Geometry: final body of the model. Coordinates: model frame, mm. Face numbers are marked on the shaded views. A direction names the side the tool comes from. Round coordinates to 2 decimals unless told otherwise and drop trailing zeros. Loops run counter-clockwise (first coordinate to the right, second up) from the corner with the lowest first, then second, coordinate; pieces in that order, holes last. Notation, with made-up numbers: M 15,51.25 L 49,51.25 A34 ccw 49,84.25 Z; hole C 83,-17 d5. An arc over 180 degrees is marked long. Answer as a JSON object with one key per item and string values.
from build123d import *

# Parameters (mm, degrees)
F1_DEPTH = 25.4
F2_R     = 7.6978943935
F3_DEPTH = 25.4
F5_DEPTH = 25.4
F7_DEPTH = 12.7
F9_DEPTH = 12.7


with BuildPart() as f1:
    # F0 (on Front) → F1 (new body)
    with BuildSketch(Plane.XZ):
        Polygon((-11.8255742339, 38.1), (-37.2255742339, 38.1), (-37.2255742339, 0), (32.6244257661, 0), (32.6244257661, 12.7), (-11.8255742339, 12.7), align=None)
    extrude(amount=F1_DEPTH)

    # F2 (on face) → F3 (cut)
    with BuildSketch(Plane.XZ.offset(25.4)):
        with Locations((-24.5255742339, 25.4)):
            Circle(F2_R)
    extrude(amount=-F3_DEPTH, mode=Mode.SUBTRACT)

    # F4 (on face) → F5 (cut)
    with BuildSketch(Plane.XZ.offset(25.4)):
        with BuildLine():
            ThreePointArc((-37.2255742339, 30.0844254155), (-34.376772158, 35.2511979241), (-29.2099996494, 38.1))
            Line((-29.2099996494, 38.1), (-37.2255742339, 38.1))
            Line((-37.2255742339, 38.1), (-37.2255742339, 30.0844254155))
        make_face()
        with BuildLine():
            Line((-11.8255742339, 38.1), (-20.5647205525, 38.1))
            ThreePointArc((-20.5647205525, 38.1), (-14.8369913494, 35.0885828844), (-11.8255742339, 29.3608536814))
            Line((-11.8255742339, 29.3608536814), (-11.8255742339, 38.1))
        make_face()
    extrude(amount=-F5_DEPTH, mode=Mode.SUBTRACT)

    # F6 (on face) → F7 (cut)
    with BuildSketch(Plane.XY.offset(12.7)):
        with BuildLine():
            ThreePointArc((26.2744257661, -12.7), (24.4145538267, -8.2098719395), (19.9244257661, -6.35))
            ThreePointArc((19.9244257661, -6.35), (13.5744257661, -12.7), (19.9244257661, -19.05))
            ThreePointArc((19.9244257661, -19.05), (24.4145538267, -17.1901280605), (26.2744257661, -12.7))
        make_face()
        with BuildLine():
            ThreePointArc((0.8744257661, -6.35), (5.3645538267, -8.2098719395), (7.2244257661, -12.7))
            ThreePointArc((7.2244257661, -12.7), (5.3645538267, -17.1901280605), (0.8744257661, -19.05))
            Line((0.8744257661, -19.05), (19.9244257661, -19.05))
            ThreePointArc((19.9244257661, -19.05), (13.5744257661, -12.7), (19.9244257661, -6.35))
            Line((19.9244257661, -6.35), (0.8744257661, -6.35))
        make_face()
        with BuildLine():
            ThreePointArc((0.8744257661, -19.05), (5.3645538267, -17.1901280605), (7.2244257661, -12.7))
            ThreePointArc((7.2244257661, -12.7), (5.3645538267, -8.2098719395), (0.8744257661, -6.35))
            ThreePointArc((0.8744257661, -6.35), (-5.4755742339, -12.7), (0.8744257661, -19.05))
        make_face()
    extrude(amount=-F7_DEPTH, mode=Mode.SUBTRACT)

    # F8 (on face) → F9 (cut)
    with BuildSketch(Plane.XY.offset(12.7)):
        with BuildLine():
            ThreePointArc((26.2291806882, 0), (30.1864649562, -2.4379608099), (32.6244257661, -6.3952450779))
            Line((32.6244257661, -6.3952450779), (32.6244257661, 0))
            Line((32.6244257661, 0), (26.2291806882, 0))
        make_face()
        with BuildLine():
            Line((32.6244257661, -25.4), (32.6244257661, -17.6856669089))
            ThreePointArc((32.6244257661, -17.6856669089), (29.8469452005, -22.6225194344), (24.910092675, -25.4))
            Line((24.910092675, -25.4), (32.6244257661, -25.4))
        make_face()
    extrude(amount=-F9_DEPTH, mode=Mode.SUBTRACT)


solid = f1.part
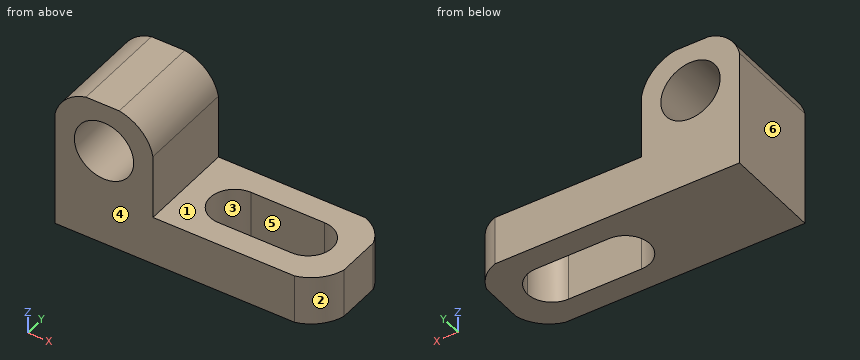
1) Section query C-C (x = 18). Return the cut outline in (y, z).
Results:
{"outline": "M -25.4,0 L -19.05,0 L -19.05,12.7 L -25.4,12.7 Z; M -6.35,0 L 0,0 L 0,12.7 L -6.35,12.7 Z"}
2) Pin query (flat end, axial travel): P1, Ø4, axis at y = -6, z = 26.5, coming from the +X side; P2, Ø9, axis at x = -24.53, z = 25.4, coming from the -Y side; P3, Ø6, axis at x = -14.5, y = -17, coming from the +Z side; P4, Ø1.5, axis at x = 17.5, y = -19, coming from the +Z side. Return the tip coordinate at first contact, or that it passes through.
Results:
{"P1": "x = -11.83", "P2": "through", "P3": "z = 37.04", "P4": "z = 12.7"}
3) Ray query, line 1 (X direction, y = -8, z = 20); line 2 (X direction, y = -11.75, z = 17.5); line 3 (X direction, y = -20.75, z = 25). Return the intervals inside material, ascending.
Results:
{"line 1": "-37.23 to -30.01, -19.04 to -11.83", "line 2": "-37.23 to -11.83", "line 3": "-37.23 to -32.21, -16.84 to -11.83"}
4) Reachability of the marked faces 1, 2 and 3 from +Z, -Z, +X, -X, +Y, -Y: full face, straight path, thin tool, end or side. Return the list, or none.
Results:
{"face 1": "+Z, +X, +Y, -Y", "face 2": "+Z, -Z, +X, -Y", "face 3": "+Z, -Z"}
5) Pull-direction query (Y, two-part tool) for the marked faces 4, 5 and 6; classes: +Y half, -Y half, draft (parallel to the pull), parting line (faces both ways), or undercut.
Results:
{"face 4": "-Y half", "face 5": "undercut", "face 6": "draft"}
6) Section query B-B (y = -11). Return the cut outline in (x, z), and give its area (3 significant figures).
Results:
{"outline": "M -37.23,0 L -5.24,0 L -5.24,12.7 L -11.83,12.7 L -11.83,29.36 A10.9 ccw -20.56,38.1 L -29.21,38.1 A10.62 ccw -37.23,30.08 Z; M 26.04,0 L 32.62,0 L 32.62,12.7 L 26.04,12.7 Z; hole C -24.53,25.4 d15.4", "area": "907 mm2"}
7) Section query A-A (z = 11). Return the cut outline in (x, y).
Results:
{"outline": "M -37.23,-25.4 L 24.91,-25.4 A10.51 ccw 32.62,-17.69 L 32.62,-6.4 A10.05 ccw 26.23,0 L -37.23,0 Z; hole M 0.87,-19.05 L 19.92,-19.05 A6.35 ccw 19.92,-6.35 L 0.87,-6.35 A6.35 ccw Z"}
8) Section query D-D (z = 25.4). Return the cut outline in (x, y), and give its area (3 significant figures).
Results:
{"outline": "M -37.23,-25.4 L -32.22,-25.4 L -32.22,0 L -37.23,0 Z; M -16.83,-25.4 L -11.83,-25.4 L -11.83,0 L -16.83,0 Z", "area": "254 mm2"}
